Geometry check sheet. Reference: drawing and pictorial views, mm from the part's lowest x, y, z. Round coordinates to 2 decimals unless told otherwise and drop trailing zeros. Write each loop counter-clockwise with the first axis right and the second up, starting at its lowest first coordinate (ties: lowest second). Pieces come first, ordered by that corner, then holes. Notation, with made-up numbers: M 50,-26.5 L 83,-26.5 A32 ccw 83,-0.5 Z; hole C 85,-5 d8. An arc over 180 degrees is marked long. Answer in a Markdown table with one row per item.
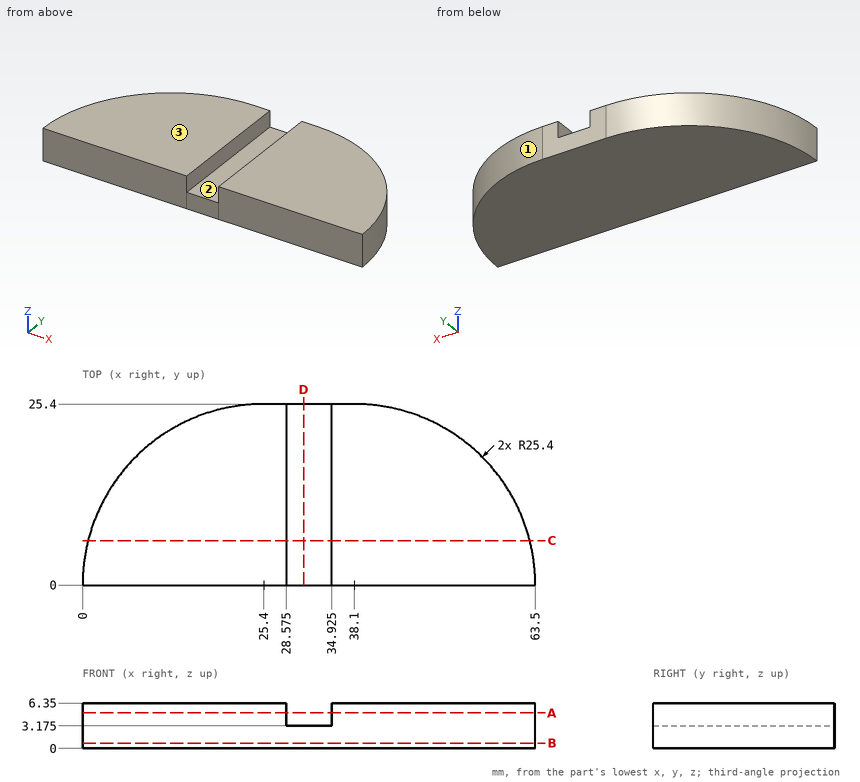
1. Go/stop test with flat-tipped pins: pin 1 (1 mm diameter, centred on y = 11.5, z = 5.5, fed in from -X); pin 2 (7 mm diameter, centred on x = 33, y = 17, fed in from +Z); pin 3 (1.5 mm diameter, centred on y = 20.5, z = 3, fed in from -X); pin 4 (3 mm diameter, centred on y = 17.5, z = 2, fed in from +X). Record where each tip stops, or that it passes through.
Found:
| item | result |
|---|---|
| pin 1 | stops at x = 2.51 |
| pin 2 | stops at z = 6.35 |
| pin 3 | stops at x = 9.43 |
| pin 4 | stops at x = 57.83 |
2. Section check C-C, the plane y = 6.25. Record the cut outline in (x, z) (3 decimals).
Found:
| item | result |
|---|---|
| outline | M 0.781,0 L 62.719,0 L 62.719,6.35 L 34.925,6.35 L 34.925,3.175 L 28.575,3.175 L 28.575,6.35 L 0.781,6.35 Z |
3. Scan lines: L1, parallel to X at y = 8.5, z = 6.25 (3 decimals); L2, parallel to X at y = 14, z = 5.75 (3 decimals); L3, parallel to Y at x = 21, z = 5.5. Record each from-to range of solid material in increasing order.
Found:
| item | result |
|---|---|
| L1 | x = 1.464 to 28.575, 34.925 to 62.036 |
| L2 | x = 4.207 to 28.575, 34.925 to 59.293 |
| L3 | y = 0 to 25.02 |
4. Section check B-B, the plane z = 0.75. Record the cut outline in (x, y) (3 decimals).
Found:
| item | result |
|---|---|
| outline | M 0,0 L 63.5,0 A25.4 ccw 38.1,25.4 L 25.4,25.4 A25.4 ccw Z |
5. Section check A-A, the plane z = 5. Record the cut outline in (x, y) (3 decimals), and give its area (3 significant figures).
Found:
| item | result |
|---|---|
| outline | M 0,0 L 28.575,0 L 28.575,25.4 L 25.4,25.4 A25.4 ccw Z; M 34.925,0 L 63.5,0 A25.4 ccw 38.1,25.4 L 34.925,25.4 Z |
| area | 1,170 mm2 |
6. Section check D-D, the plane x = 31. Record the cut outline in (y, z) (3 decimals).
Found:
| item | result |
|---|---|
| outline | M 0,0 L 25.4,0 L 25.4,3.175 L 0,3.175 Z |
7. Draft check along X on the marked faces 1, 2 and 3. Enter one of: +X half, -X half, draft (parallel to the pull), parting line (faces both ways), or undercut.
Found:
| item | result |
|---|---|
| face 1 | +X half |
| face 2 | undercut |
| face 3 | draft |
